Could you check a few things on this model? Use its own coordinates, in mm. Face numbers are marked on the shaded views. Round coordinates to 2 decimals unless told otherwise and drop trailing zeros. Loops run counter-clockwise (first coordinate to the right, second up) from the corner with the lowest first, then second, coordinate; pieces in that order, holes last. Notation, with made-up numbers: (44.5, 10.25) - (100.5, 10.25) arc R22 ccw to (100.5, 25.25) - close; hole circle Ø9 at (23.5, 52). An arc over 180 degrees is marked (long way). Use one line per item in the form item = value.
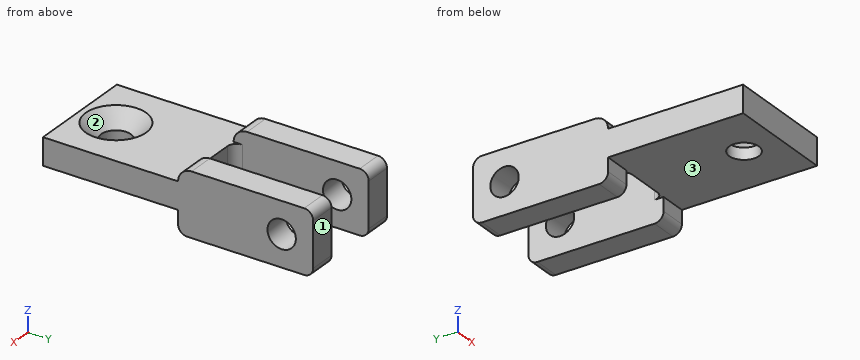
```python
from build123d import *

# Parameters (mm, degrees)
F0_W           = 3.05
F0_H           = 15
F1_DEPTH       = 3
F3_DEPTH       = 3
F6_D           = 3.3
F6_CSINK_D     = 6.72
F6_CSINK_ANGLE = 90
F8_D           = 3.15
F9_T1_DEPTH    = 3
F9_T3_DEPTH    = 8
F9_T5_DEPTH    = 8


# Not quite as in the source:
# - a fillet or chamfer that OpenCascade refuses, or shapes differently, is made with other operations: its cross-section is extruded or revolved along the edge and cut away or added


with BuildPart() as f1:
    # F0 (on Top) → F1 (new body)
    with BuildSketch(Plane.XY):
        with Locations((1.525, 7.5)):
            Rectangle(F0_W, F0_H)
    extrude(amount=F1_DEPTH)

    # F2 (on face) → F3 (join)
    with BuildSketch(Plane.YZ.offset(3.05)):
        with BuildLine():
            Line((0, 3), (0, 0))
            Line((0, 0), (15, 0))
            Line((15, 0), (15, -2.5))
            Line((15, -2.5), (30, -2.5))
            Line((30, -2.5), (30, 4.5))
            Line((30, 4.5), (16.5, 4.5))
            ThreePointArc((16.5, 4.5), (15.4393398282, 4.0606601718), (15, 3))
            Line((15, 3), (0, 3))
        make_face()
    extrude(amount=F3_DEPTH)

    # F4: F1 across face


with BuildPart() as f1_1:
    add(f1.part)
    add(f1.part.mirror(Plane(origin=(0, 7.5, 1.5), x_dir=(0, -1, 0), z_dir=(-1, 0, 0))))

    # F6 (through all)
    with Locations(Plane.XY.offset(3)):
        with Locations((0, 4)):
            CounterSinkHole(F6_D / 2, F6_CSINK_D / 2, counter_sink_angle=F6_CSINK_ANGLE)

    # F8 (through all)
    with Locations(Plane.YZ.offset(6.05)):
        with Locations((26.5, 1)):
            Hole(F8_D / 2)

    # F9: fillet of radius 1 on 8 edges, made by hand

    # F9_s2 → F9_t1 (join)
    with BuildSketch(Plane.XY):
        with BuildLine():
            ThreePointArc((2.05, 15), (2.7571067812, 15.2928932188), (3.05, 16))
            Line((3.05, 16), (3.05, 15))
            Line((3.05, 15), (2.05, 15))
        make_face()
        with BuildLine():
            ThreePointArc((-2.05, 15), (-2.7571067812, 15.2928932188), (-3.05, 16))
            Line((-3.05, 16), (-3.05, 15))
            Line((-3.05, 15), (-2.05, 15))
        make_face()
    extrude(amount=F9_T1_DEPTH)

    # F9_s4 → F9_t3 (cut)
    with BuildSketch(Plane.YZ.offset(0.55)):
        with BuildLine():
            ThreePointArc((29, 4.5), (29.7071067812, 4.2071067812), (30, 3.5))
            Line((30, 3.5), (30, 4.5))
            Line((30, 4.5), (29, 4.5))
        make_face()
        with BuildLine():
            ThreePointArc((29, -2.5), (29.7071067812, -2.2071067812), (30, -1.5))
            Line((30, -1.5), (30, -2.5))
            Line((30, -2.5), (29, -2.5))
        make_face()
        with BuildLine():
            ThreePointArc((15, -1.5), (15.2928932188, -2.2071067812), (16, -2.5))
            Line((16, -2.5), (15, -2.5))
            Line((15, -2.5), (15, -1.5))
        make_face()
    extrude(amount=F9_T3_DEPTH, mode=Mode.SUBTRACT)

    # F9_s6 → F9_t5 (cut)
    with BuildSketch(Plane.YZ.offset(-8.55)):
        with BuildLine():
            ThreePointArc((29, 4.5), (29.7071067812, 4.2071067812), (30, 3.5))
            Line((30, 3.5), (30, 4.5))
            Line((30, 4.5), (29, 4.5))
        make_face()
        with BuildLine():
            ThreePointArc((29, -2.5), (29.7071067812, -2.2071067812), (30, -1.5))
            Line((30, -1.5), (30, -2.5))
            Line((30, -2.5), (29, -2.5))
        make_face()
        with BuildLine():
            ThreePointArc((15, -1.5), (15.2928932188, -2.2071067812), (16, -2.5))
            Line((16, -2.5), (15, -2.5))
            Line((15, -2.5), (15, -1.5))
        make_face()
    extrude(amount=F9_T5_DEPTH, mode=Mode.SUBTRACT)


solid = f1_1.part
```
1. If we section it at B-B, the plane z = 1: Write out the boundary of the cut face in (x, y) (3 decimals), plus the area to 3 significant figures.
Solution:
outline = (-6.05, 0) - (6.05, 0) - (6.05, 24.925) - (3.05, 24.925) - (3.05, 16) arc R1 cw to (2.05, 15) - (-2.05, 15) arc R1 cw to (-3.05, 16) - (-3.05, 24.925) - (-6.05, 24.925) - close; (-6.05, 28.075) - (-3.05, 28.075) - (-3.05, 30) - (-6.05, 30) - close; (3.05, 28.075) - (6.05, 28.075) - (6.05, 30) - (3.05, 30) - close; hole circle Ø3.3 at (0, 4)
area = 244 mm^2
2. If we section it at D-D, the plane y = 21.25: Write out the boundary of the cut face in (x, z).
Solution:
outline = (-6.05, -2.5) - (-3.05, -2.5) - (-3.05, 4.5) - (-6.05, 4.5) - close; (3.05, -2.5) - (6.05, -2.5) - (6.05, 4.5) - (3.05, 4.5) - close
3. Please list where these lines run through material, in increasing order: line 1 along X through (y, z) = (23, -0.5); line 2 along Z through (x, y) = (3.75, 26.5) (3 decimals); line 3 along X through (y, z) = (4, 0.45).
Solution:
line_1 = -6.05 to -3.05, 3.05 to 6.05
line_2 = -2.5 to -0.575, 2.575 to 4.5
line_3 = -6.05 to -1.65, 1.65 to 6.05
4. If we section it at C-C, the plane x = -4.25: Write out the boundary of the cut face in (y, z) (3 decimals), plus the area to 3 significant figures.
Solution:
outline = (0, 0) - (15, 0) - (15, -1.5) arc R1 ccw to (16, -2.5) - (29, -2.5) arc R1 ccw to (30, -1.5) - (30, 3.5) arc R1 ccw to (29, 4.5) - (16.5, 4.5) arc R1.5 ccw to (15, 3) - (0, 3) - close; hole circle Ø3.15 at (26.5, 1)
area = 141 mm^2
5. We'd pull the mould along Y, two halves only. Please class the marked faces 1, 2 and 3: +Y half, -Y half, draft (parallel to the pull), parting line (faces both ways), or undercut.
Solution:
face_1 = +Y half
face_2 = undercut
face_3 = draft
6. If we section it at A-A, the plane x = 0: Write out the boundary of the cut face in (y, z).
Solution:
outline = (0, 0) - (2.35, 0) - (2.35, 1.29) - (0.64, 3) - (0, 3) - close; (5.65, 0) - (15, 0) - (15, 3) - (7.36, 3) - (5.65, 1.29) - close
7. For P1, Ø1, axis at x = 3, z = -1, coming from the +Y side; P2, Ø0.8, axis at x = 5, z = -0.5, coming from the -Y side; P3, Ø1.5, axis at x = 2, y = 10.5, coming from the -Z side; P4, Ø6, axis at x = -2, y = 6.5, coming from the +Z side, each with a flat end and sliding along its axis, tell me the tip position at first contact or that it passes through.
Solution:
P1 = 30
P2 = 15
P3 = 0
P4 = 3
